For this review, take the finished solid that the model builds, in its own axes (mm). Coordinates: 2 decimals unless noted, no trailing zeros. Loops run counter-clockwise (first coordinate to the right, second up) from the corner with the lowest first, then second, coordinate; pieces in that order, holes last.
1. To check wall thickness, follow probe 1 along X at (y, z) = (4.5, 9); probe 2 along X at (y, z) = (6, 9); probe 3 along Y at (x, z) = (-146.5, 9.75). State the ranges of each line that lie inside material, in increasing order.
2. Take a section at A-A, the plane y = 2.75. State the section outline as (x, z) points.
3. Mouldability with a two-part tool opening along Z and no side actions: class faces 1 (the face through (0, 2, 9)), 2 (the face through (-178.98, 4.93, 8.41)), 3 (the face through (-31.278, 2.535, 7.334)) as pulls with the +Z half, pulls with the -Z half, needs draft (parallel to the pull), parting line crosses it, or undercut.
4. Take a section at B-B, the plane x = -30. State the section outline as (y, z) points.
5. Clearance check with flat-ended pins moving along their axes: P1, Ø1, axis at y = 3.5, z = 8, coming from the -X side; P2, Ø1.5, axis at x = -45, z = 14.5, coming from the +Y side; P3, Ø4, axis at x = -129, z = 4, coming from the -Y side. State where each tip first meets the part, or that it passes through.
```python
from build123d import *

# Parameters (mm, degrees)
BOSS_EXTRUDE1_DEPTH = 5
SKETCH2_R           = 9
BOSS_EXTRUDE2_DEPTH = 5
SKETCH3_R           = 5.5
CUT_EXTRUDE1_DEPTH  = 181.18046509
SKETCH4_R           = 2.1
CUT_EXTRUDE2_DEPTH  = 180.972220079


with BuildPart() as part:
    # Sketch1 → Boss-Extrude1 (new body)
    with BuildSketch(Plane(origin=(0, 0, 0), x_dir=(1, 0, 0), z_dir=(0, 1, 0))):
        with BuildLine():
            Line((0, 0), (-170, 0))
            ThreePointArc((-170, 0), (-179, -9), (-170, -18))
            Line((-170, -18), (0, -18))
            Line((0, -18), (0, 0))
        make_face()
    extrude(amount=BOSS_EXTRUDE1_DEPTH)

    # Sketch2 → Boss-Extrude2 (add)
    with BuildSketch(Plane(origin=(0, 5, 0), x_dir=(1, 0, 0), z_dir=(0, 1, 0))):
        with Locations(Location((-170, -9, 0), (0, 0, 270))):
            Circle(SKETCH2_R)
    extrude(amount=BOSS_EXTRUDE2_DEPTH)

    # Sketch3 → Cut-Extrude1 (cut, through all)
    with BuildSketch(Plane(origin=(0, 10, 0), x_dir=(1, 0, 0), z_dir=(0, 1, 0))):
        with Locations(Location((-170, -9, 0), (0, 0, 270))):
            Circle(SKETCH3_R)
    extrude(amount=-CUT_EXTRUDE1_DEPTH, mode=Mode.SUBTRACT)

    # Sketch4 → Cut-Extrude2 (cut, through all)
    with BuildSketch(Plane(origin=(0, 5, 0), x_dir=(1, 0, 0), z_dir=(0, 1, 0))):
        with Locations(Location((-10, -9, 0), (0, 0, 270))):
            Circle(SKETCH4_R)
        with Locations(Location((-30, -9, 0), (0, 0, 270))):
            Circle(SKETCH4_R)
    extrude(amount=-CUT_EXTRUDE2_DEPTH, mode=Mode.SUBTRACT)


solid = part.part
```
Results list:
1. probe 1: x = -179 to -175.5, -164.5 to -32.1, -27.9 to -12.1, -7.9 to 0
1. probe 2: x = -179 to -175.5, -164.5 to -161
1. probe 3: y = 0 to 5
2. outline: (-170, 0) - (0, 0) - (0, 18) - (-170, 18) arc R9 ccw to start; hole circle Ø11 at (-170, 9); hole circle Ø4.2 at (-30, 9); hole circle Ø4.2 at (-10, 9)
3. face 1: needs draft
3. face 2: parting line crosses it
3. face 3: undercut
4. outline: (0, 0) - (5, 0) - (5, 6.9) - (0, 6.9) - close; (0, 11.1) - (5, 11.1) - (5, 18) - (0, 18) - close
5. P1: stops at x = -178.99
5. P2: stops at y = 5
5. P3: stops at y = 0
